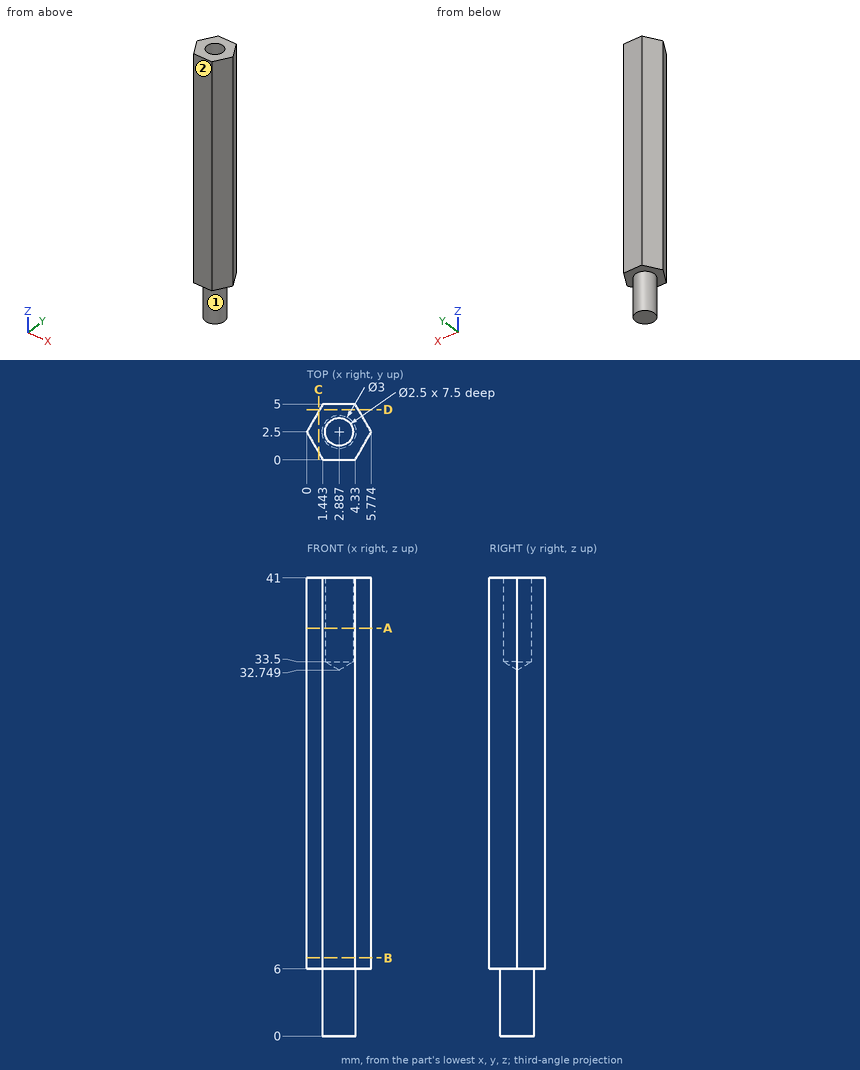
Verification items for this drawing (mm, ordinates from the low corner). A direction names the side the tool comes from. Give positions to 0.01 mm unless a question says otherwise; leave off trailing zeros. Write each loop counter-clockwise with the first axis right and the second up, starting at its lowest first coordinate (ties: lowest second). Pieces come first, ordered by that corner, then holes.
1) Access from +Z, -Z, +X, -X, +Y, -Y to the whole of each face (thin tool, end or side, straight path). Record for the marked faces 1 and 2.
2) Gauge pin test, flat end, axial feed: pin 1 (2 mm diameter, centred on x = 0.5, y = 3.5, fed in from +Z). Record the tip position at first contact, or that the pin passes through.
3) Section check D-D, the plane y = 4.5. Record the boundary of the cut face in (x, z) (1 decimal).
4) Material ranges on L1, parallel to Z at x = 5.35, y = 1.9; L2, parallel to X at y = 3.4, z = 38 (1 decimal); L3, parallel to Y at x = 4, z = 34 (1 decimal), recorded low to high.
5) Section check B-B, the plane z = 7. Record the boundary of the cut face in (x, y).
6) Section check A-A, the plane z = 36.5. Record the boundary of the cut face in (x, y).
7) Section check C-C, the plane x = 1.05. Record the boundary of the cut face in (y, z).
Computed:
1. face 1: -Z
1. face 2: +Z, -Z, +X, -X, -Y
2. pin 1: stops at z = 41
3. outline: (1.2, 6) - (4.6, 6) - (4.6, 41) - (1.2, 41) - close
4. L1: z = 6 to 41
4. L2: x = 0.5 to 2, 3.8 to 5.3
4. L3: y = 0 to 1.9, 3.1 to 5
5. outline: (0, 2.5) - (1.44, 0) - (4.33, 0) - (5.77, 2.5) - (4.33, 5) - (1.44, 5) - close
6. outline: (0, 2.5) - (1.44, 0) - (4.33, 0) - (5.77, 2.5) - (4.33, 5) - (1.44, 5) - close; hole circle Ø2.5 at (2.89, 2.5)
7. outline: (0.68, 6) - (4.32, 6) - (4.32, 41) - (0.68, 41) - close
